Part print with two shaded views. Sizes in mm from the minimum x, y, z corner. A direction names the side the tool comes from. Round coordinates to 2 decimals unless told otherwise and drop trailing zeros. Write each loop counter-clockwise with the first axis right and the second up, starting at its lowest first coordinate (ties: lowest second). Pieces come first, ordered by that corner, then holes. Notation, with made-up numbers: (43.5, 7) -> (58.5, 7) arc R15 cw to (58.5, 19) -> close; hole circle Ø7 at (24.25, 31.5). An arc over 180 degrees is marked (long way). Put each result on its own line as item: value. Start each with the question number.
1. Pull direction X, two halves, no side cores. Call the marked faces 1, 2, 3 and 4: pulls with the +X half, pulls with the -X half, needs draft (parallel to the pull), parting line crosses it, or undercut.
2. Saw through at A-A on y = 50.8. List the corners of the cut face in (x, z), and give its area (3 significant figures).
3. 3-axis set-ups, long thin cutter, end or side, ignore diameter. For the marked faces 5, 6 and 7: which of +Z, -Z, +X, -X, +Y, -Y reach the whole face in a straight line?
4. Saw through at B-B on x = 38.1. List the corners of the cut face in (y, z).
5. Saw through at C-C on z = 62. List the corners of the cut face in (x, y).
6. Flat gauge pins, fed straight in: P1, Ø3.5, axis at x = 8, y = 38, coming from the -Z side; P2, Ø1.4, axis at y = 46, z = 1, coming from the -X side; P3, Ø5, axis at x = 47.5, z = 60.5, coming from the -Y side. Where does each tip first touch, or does it go through?
7. Drill centre lines: line 1 (Y direction, x = 38.1, z = 42.5); line 2 (X direction, y = 50, z = 23) (1 decimal); line 3 (Y direction, x = 38.1, z = 47.5). Where is each one in solid material? Low to high. Write a range as from..to.
8. Saw through at D-D on x = 95. List the corners of the cut face in (y, z), and give its area (3 significant figures).
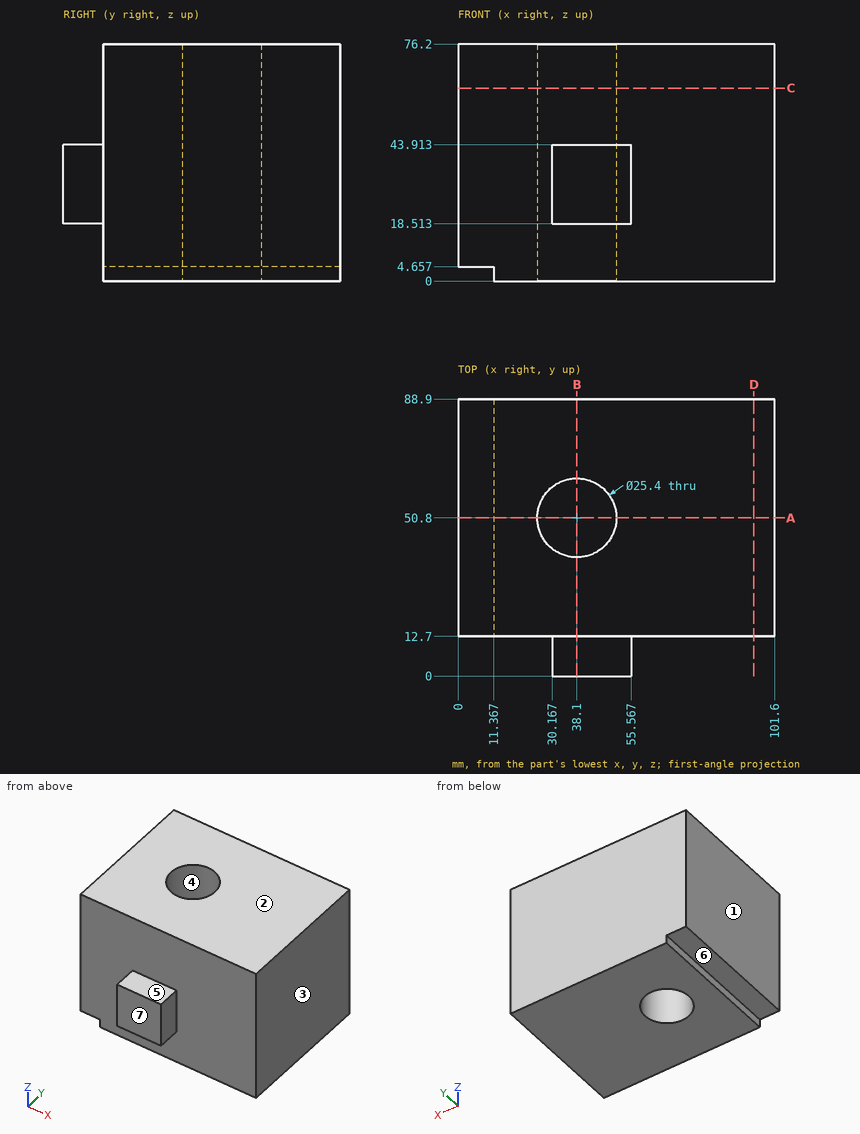
Return value:
1. face 1: pulls with the -X half
1. face 2: needs draft
1. face 3: pulls with the +X half
1. face 4: undercut
2. outline: (0, 4.66) -> (11.37, 4.66) -> (11.37, 0) -> (25.4, 0) -> (25.4, 76.2) -> (0, 76.2) -> close; (50.8, 0) -> (101.6, 0) -> (101.6, 76.2) -> (50.8, 76.2) -> close
2. area: 5,750 mm^2
3. face 5: +Z, +X, -X, -Y
3. face 6: -Z, -X, +Y, -Y
3. face 7: +Z, -Z, +X, -X, -Y
4. outline: (0, 18.51) -> (12.7, 18.51) -> (12.7, 0) -> (38.1, 0) -> (38.1, 76.2) -> (12.7, 76.2) -> (12.7, 43.91) -> (0, 43.91) -> close; (63.5, 0) -> (88.9, 0) -> (88.9, 76.2) -> (63.5, 76.2) -> close
5. outline: (0, 12.7) -> (101.6, 12.7) -> (101.6, 88.9) -> (0, 88.9) -> close; hole circle Ø25.4 at (38.1, 50.8)
6. P1: stops at z = 4.66
6. P2: stops at x = 11.37
6. P3: stops at y = 12.7
7. line 1: y = 0..38.1, 63.5..88.9
7. line 2: x = 0..25.4, 50.8..101.6
7. line 3: y = 12.7..38.1, 63.5..88.9
8. outline: (12.7, 0) -> (88.9, 0) -> (88.9, 76.2) -> (12.7, 76.2) -> close
8. area: 5,810 mm^2
